```python
from build123d import *

# Parameters (mm, degrees)
F1_DEPTH = 6.35
F2_R     = 6.3499
F0_R     = 5.08
F3_DEPTH = 6.35
F4_DEPTH = 6.35


# Not quite as in the source:
# - a fillet or chamfer is up to 0.001 mm smaller than in the source, because OpenCascade refuses the exact size


with BuildPart() as f1:
    # F0 (on Front) → F1 (new body, symmetric)
    with BuildSketch(Plane.XZ):
        with BuildLine():
            Line((9.525, 6.35), (-9.525, 6.35))
            Line((-9.525, 6.35), (-9.525, -6.35))
            Line((-9.525, -6.35), (9.525, -6.35))
            ThreePointArc((9.525, -6.35), (7.296147458, 0), (9.525, 6.35))
        make_face()
        with BuildLine():
            Line((-9.525, -6.35), (-9.525, 6.35))
            ThreePointArc((-9.525, 6.35), (-15.875, 0), (-9.525, -6.35))
        make_face()
    extrude(amount=F1_DEPTH, both=True)

    # F2 (radius 6.35 in the source; OpenCascade refuses exactly that, so slightly less here)
    f2_edges = [f1.edges().sort_by_distance(p)[0] for p in [
        (0, -6.35, 6.35),
        (0, 6.35, 6.35),
        (0, -6.35, -6.35),
        (0, 6.35, -6.35),
    ]]
    fillet(f2_edges, radius=F2_R)

    # F0 (on Front) → F3 (join)
    with BuildSketch(Plane.XZ):
        with BuildLine():
            ThreePointArc((27.616147458, 0), (20.8210502669, 9.5866067556), (9.525, 6.35))
            Line((9.525, 6.35), (9.525, -6.35))
            ThreePointArc((9.525, -6.35), (20.8210502669, -9.5866067556), (27.616147458, 0))
        make_face()
        with Locations((17.456147458, 0)):
            Circle(F0_R, mode=Mode.SUBTRACT)
        with BuildLine():
            Line((9.525, -6.35), (9.525, 6.35))
            ThreePointArc((9.525, 6.35), (7.296147458, 0), (9.525, -6.35))
        make_face()
    extrude(amount=F3_DEPTH)

    # F0 (on Front) → F4 (join, symmetric)
    with BuildSketch(Plane.XZ):
        with Locations((17.456147458, 0)):
            Circle(F0_R)
    extrude(amount=F4_DEPTH, both=True)


solid = f1.part
```
The listing builds one solid part. Answer for the finished solid, in the listing's coordinates (mm). A direction names the side the tool comes from. Give positions to 0.01 mm unless a question says otherwise; leave off trailing zeros. Loops run counter-clockwise (first coordinate to the right, second up) from the corner with the lowest first, then second, coordinate; pieces in that order, holes last. Notation, with made-up numbers: (38.25, 3.5) - (71.25, 3.5) arc R18 ccw to (71.25, 23.5) - close; hole circle Ø4 at (-10, -33.75). An arc over 180 degrees is marked (long way). Answer as CSV lines item,"result". Start each with the question number.
Item 1: A cutting plane is placed at D-D on z = -8. Determine the outline of the cut face in (x, y), then the cut area to 3 significant figures.
Item 2: A cutting plane is placed at B-B on z = 7. Determine the outline of the cut face in (x, y), then the cut area to 3 significant figures.
Item 3: The mould has two halves that part along X. Classify faces 6 (the face through (0.13, -4.44, -4.54)), 7 (the face through (7.297, 2.425, -0.096)): +X half, -X half, draft (parallel to the pull), parting line (faces both ways), or undercut.
Item 4: For faces 1 (the face through (0.13, 4.44, -4.54)), 2 (the face through (-0.13, 4.44, 4.54)), 3 (the face through (17, -6.35, 0)), 4 (the face through (-0.13, -4.44, 4.54)), 5 (the face through (20, 0, 5)), determine the directions among +Z, -Z, +X, -X, +Y, -Y from which every point of the face is accessible in a straight line to the end or side of a thin tool.
Item 5: Each of these flat-tipped pins is pushed along its axis until it touches: pin 1 (1.5 mm diameter, centred on y = -3, z = -2, fed in from -X); pin 2 (3 mm diameter, centred on x = 4, y = 1.5, fed in from -Z); pin 3 (5 mm diameter, centred on x = 9, z = 5.5, fed in from +Y); pin 4 (3 mm diameter, centred on x = -0.5, z = 0.5, fed in from +Y). Where does it stop, or does it pass through?
Item 6: A cutting plane is placed at C-C on x = 16. Determine the outline of the cut face in (y, z), then the cut area to 3 significant figures.
Item 7: Find the intervals of material crossed by line 1 (X direction, y = 4, z = 2); line 2 (Y direction, x = -5.5, z = -5.25), in increasing order. Write a range as from..to.
Found:
1,outline,"(11.19, -6.35) - (23.72, -6.35) - (23.72, 0) - (11.19, 0) - close"
1,area,"79.5 mm^2"
2,outline,"(10.09, -6.35) - (24.82, -6.35) - (24.82, 0) - (10.09, 0) - close"
2,area,"93.5 mm^2"
3,face 6,"draft"
3,face 7,"undercut"
4,face 1,"-Z, -X, +Y"
4,face 2,"+Z, -X, +Y"
4,face 3,"+Z, -Z, +X, -X, -Y"
4,face 4,"+Z, -X, -Y"
4,face 5,"+Y"
5,pin 1,"stops at x = -15.2"
5,pin 2,"stops at z = -6.35"
5,pin 3,"stops at y = 5.43"
5,pin 4,"stops at y = 6.35"
6,outline,"(-6.35, -10.06) - (0, -10.06) - (0, -4.87) - (6.35, -4.87) - (6.35, 4.87) - (0, 4.87) - (0, 10.06) - (-6.35, 10.06) - close"
6,area,"190 mm^2"
7,line 1,"x = -14.03..7.49, 12.79..22.13"
7,line 2,"y = -3.57..3.57"
